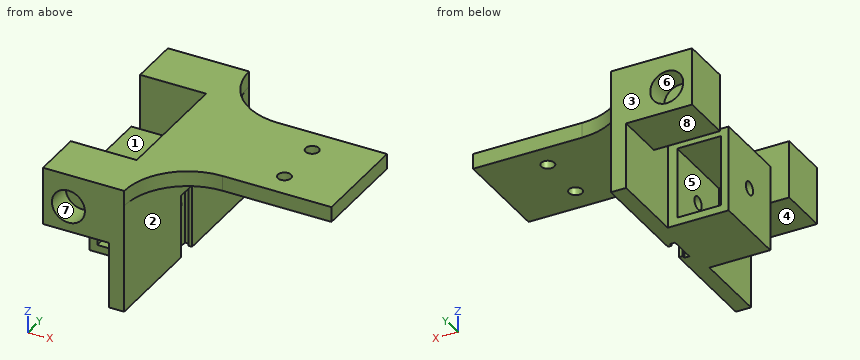
```python
from build123d import *

# Parameters (mm, degrees)
SKETCH1_W               = 74
SKETCH1_H               = 90
SKETCH1_R               = 2.6
BOSS_EXTRUDE1_DEPTH     = 6
SKETCH2_W               = 6
SKETCH2_H               = 90
BOSS_EXTRUDE2_DEPTH     = 43
SKETCH4_W               = 68
SKETCH4_H               = 25
CUT_EXTRUDE3_DEPTH      = 6
FILLET2_R               = 25
SKETCH5_W               = 34
SKETCH5_H               = 30
BOSS_EXTRUDE3_DEPTH     = 24
CUT_EXTRUDE1_DEPTH      = 125.197423484
CUT_EXTRUDE1_DEPTH_BACK = 125.197423484
SKETCH3_R               = 2.6
SKETCH6_W               = 17.25
SKETCH6_H               = 28
CUT_EXTRUDE4_DEPTH      = 105.522724802
CUT_EXTRUDE5_DEPTH      = 25
SKETCH8_W               = 22.83
SKETCH8_H               = 20
BOSS_EXTRUDE4_DEPTH     = 26
SKETCH9_R               = 6.5
CUT_EXTRUDE6_DEPTH      = 10
CUT_EXTRUDE7_START      = -10
SKETCH10_R              = 6.5
CUT_EXTRUDE7_DEPTH      = 10


with BuildPart() as part:
    # Sketch1 → Boss-Extrude1 (new body)
    with BuildSketch(Plane.XY):
        with Locations((37, 45)):
            Rectangle(SKETCH1_W, SKETCH1_H)
        with Locations((50, 55)):
            Circle(SKETCH1_R, mode=Mode.SUBTRACT)
        with Locations((50, 35)):
            Circle(SKETCH1_R, mode=Mode.SUBTRACT)
    extrude(amount=BOSS_EXTRUDE1_DEPTH)

    # Sketch2 → Boss-Extrude2 (add)
    with BuildSketch(Plane(origin=(0, 0, 0), x_dir=(-1, 0, 0), z_dir=(0, 0, -1))):
        with Locations((-3, 45)):
            Rectangle(SKETCH2_W, SKETCH2_H)
    extrude(amount=BOSS_EXTRUDE2_DEPTH)

    # Sketch4 → Cut-Extrude3 (cut)
    with BuildSketch(Plane(origin=(0, 0, 0), x_dir=(-1, 0, 0), z_dir=(0, 0, -1))):
        with Locations((-40, 77.5)):
            Rectangle(SKETCH4_W, SKETCH4_H)
        with Locations((-40, 12.5)):
            Rectangle(SKETCH4_W, SKETCH4_H)
    extrude(amount=-CUT_EXTRUDE3_DEPTH, mode=Mode.SUBTRACT)

    # Fillet2
    fillet2_edges = [part.edges().sort_by_distance(p)[0] for p in [
        (6, 65, 3),
        (6, 25, 3),
    ]]
    fillet(fillet2_edges, radius=FILLET2_R - 0.0001)  # a hair under: the kernel refuses the full size

    # Sketch5 → Boss-Extrude3 (add)
    with BuildSketch(Plane.ZY):
        with Locations((-26, 45)):
            Rectangle(SKETCH5_W, SKETCH5_H)
    extrude(amount=BOSS_EXTRUDE3_DEPTH)

    # Sketch3 → Cut-Extrude1 (cut, two sides: drawn at the far end of the back side and taken through both)
    with BuildSketch(Plane.ZY.offset(-CUT_EXTRUDE1_DEPTH_BACK)):
        with Locations((-26, 45)):
            Circle(SKETCH3_R)
    extrude(amount=CUT_EXTRUDE1_DEPTH + CUT_EXTRUDE1_DEPTH_BACK, mode=Mode.SUBTRACT)

    # Sketch6 → Cut-Extrude4 (cut, through all)
    with BuildSketch(Plane(origin=(0, 60, 0), x_dir=(1, 0, 0), z_dir=(0, 1, 0))):
        with Locations((-12.375, 26)):
            Rectangle(SKETCH6_W, SKETCH6_H)
    extrude(amount=-CUT_EXTRUDE4_DEPTH, mode=Mode.SUBTRACT)

    # Sketch7 → Cut-Extrude5 (cut)
    with BuildSketch(Plane(origin=(0, 0, -43), x_dir=(-1, 0, 0), z_dir=(0, 0, -1))):
        Polygon((-2.5, 50.15), (-4.5, 50.15), (-4.5, 48.9), (-7.5, 48.9), (-7.5, 41.1), (-4.5, 41.1), (-4.5, 39.85), (-2.5, 39.85), align=None)
    extrude(amount=-CUT_EXTRUDE5_DEPTH, mode=Mode.SUBTRACT)

    # Sketch8 → Boss-Extrude4 (add)
    with BuildSketch(Plane.ZY):
        with Locations((-5.415, 10)):
            Rectangle(SKETCH8_W, SKETCH8_H)
        with Locations((-5.415, 80)):
            Rectangle(SKETCH8_W, SKETCH8_H)
    extrude(amount=BOSS_EXTRUDE4_DEPTH)

    # Sketch9 → Cut-Extrude6 (cut)
    with BuildSketch(Plane.XZ):
        with Locations(Location((-16, -6.83, 0), (0, 0, 270))):
            Circle(SKETCH9_R)
    extrude(amount=-CUT_EXTRUDE6_DEPTH, mode=Mode.SUBTRACT)

    # Sketch10 → Cut-Extrude7 (cut)
    with BuildSketch(Plane(origin=(0, 90, 0), x_dir=(1, 0, 0), z_dir=(0, 1, 0)).offset(CUT_EXTRUDE7_START)):
        with Locations(Location((-16, 6.83, 0), (0, 0, 90))):
            Circle(SKETCH10_R)
    extrude(amount=CUT_EXTRUDE7_DEPTH, mode=Mode.SUBTRACT)


solid = part.part
```
Here's how the part is built. I have some questions about the finished solid (model axes, mm). Face numbers are marked on the shaded views. A direction names the side the tool comes from. Coordinates: 2 decimals unless noted, no trailing zeros. Loops run counter-clockwise (first coordinate to the right, second up) from the corner with the lowest first, then second, coordinate; pieces in that order, holes last. Notation, with made-up numbers: (54.5, 69) - (60.5, 69) arc R23 ccw to (60.5, 108) - close; hole circle Ø7 at (39.25, 9.25). An arc over 180 degrees is marked (long way). Return JSON: item names as keys, results as strings. Group by question number.
Item 1: If we section it at B-B on z = -26: Write out the boundary of the cut face in (x, y), and give its area (3 significant figures).
Item 2: If we section it at C-C on x = -1.5: Write out the boundary of the cut face in (y, z).
Item 3: If we section it at A-A on y = 55: Write out the boundary of the cut face in (x, z).
Item 4: Will these pins go through, and if not, where does the flat tip stop? P1, Ø0.6, axis at y = 50, z = -36.5, coming from the -X side; P2, Ø5, axis at y = 39.5, z = -28.5, coming from the +X side; P3, Ø3, axis at y = 45.5, z = -34, coming from the +X side.
Item 5: If we section it at D-D on y = 45: Write out the boundary of the cut face in (x, z).
Item 6: I need wall thicknesses on line 1 (Y direction, x = 50, z = 4); line 2 (Y direction, x = -9.5, z = -11); line 3 (X direction, y = 48, z = -34). Which ranges of each line are inside material? Lowest first, please. Write a range as from..to.
Item 7: On a 3-axis mill with a long thin cutter (end or side, diameter ignored), from which of +Z, -Z, +X, -X, +Y, -Y can I reach the whole of each face in a straight line? I mean the marked faces 4, 5, 6, 7 and 8. Say none if no direction works.
Item 8: We'd pull the mould along Y, two halves only. Please class the marked faces 1, 2 and 3: +Y half, -Y half, draft (parallel to the pull), parting line (faces both ways), or undercut.
Calculated:
{
 "1": {"outline": "(-24, 30) - (-21, 30) - (-21, 42.4) - (-24, 42.4) - close; (-24, 47.6) - (-21, 47.6) - (-21, 60) - (-24, 60) - close; (-3.75, 30) - (0, 30) - (0, 0) - (6, 0) - (6, 41.1) - (4.5, 41.1) - (4.5, 39.85) - (2.5, 39.85) - (2.5, 42.4) - (-3.75, 42.4) - close; (-3.75, 47.6) - (2.5, 47.6) - (2.5, 50.15) - (4.5, 50.15) - (4.5, 48.9) - (6, 48.9) - (6, 90) - (0, 90) - (0, 60) - (-3.75, 60) - close", "area": "662 mm^2"},
 "2": {"outline": "(0, -16.83) - (20, -16.83) - (20, 6) - (0, 6) - close; (30, -43) - (60, -43) - (60, -9) - (30, -9) - close; (70, -16.83) - (90, -16.83) - (90, 6) - (70, 6) - close; hole circle Ø5.2 at (45, -26)"},
 "3": {"outline": "(-24, -43) - (6, -43) - (6, 0) - (47.4, 0) - (47.4, 6) - (0, 6) - (0, -9) - (-24, -9) - close; (52.6, 0) - (74, 0) - (74, 6) - (52.6, 6) - close; hole (-21, -40) - (-3.75, -40) - (-3.75, -12) - (-21, -12) - close"},
 "4": {"P1": "stops at x = -24", "P2": "stops at x = 6", "P3": "stops at x = 2.5"},
 "5": {"outline": "(-24, -43) - (2.5, -43) - (2.5, -28.6) - (-3.75, -28.6) - (-3.75, -40) - (-21, -40) - (-21, -28.6) - (-24, -28.6) - close; (-24, -23.4) - (-21, -23.4) - (-21, -12) - (-3.75, -12) - (-3.75, -23.4) - (2.5, -23.4) - (2.5, -18) - (6, -18) - (6, 0) - (74, 0) - (74, 6) - (0, 6) - (0, -9) - (-24, -9) - close"},
 "6": {"line 1": "y = 25..32.4, 37.6..52.4, 57.6..65", "line 2": "y = 0..20, 30..60, 70..90", "line 3": "x = -24..-21, -3.75..2.5"},
 "7": {"face 4": "-Z, -X, -Y", "face 5": "none", "face 6": "+Y", "face 7": "-Y", "face 8": "-Z, -X, +Y"},
 "8": {"face 1": "undercut", "face 2": "draft", "face 3": "+Y half"}
}
